from build123d import *

# Parameters (mm, degrees)
SKETCH1_W           = 50
SKETCH1_H           = 50
BOSS_EXTRUDE1_DEPTH = 0.8
FILLET1_R           = 5
SKETCH2_R           = 2
CUT_EXTRUDE1_DEPTH  = 36.364388868
SKETCH3_R           = 19.807187389
BOSS_EXTRUDE2_DEPTH = 1.5
SKETCH4_R           = 17.5
CUT_EXTRUDE2_DEPTH  = 1.5
SKETCH6_R           = 10
CUT_EXTRUDE3_DEPTH  = 36.387144558


with BuildPart() as part:
    # Sketch1 → Boss-Extrude1 (new body)
    with BuildSketch(Plane.XY):
        Rectangle(SKETCH1_W, SKETCH1_H)
    extrude(amount=BOSS_EXTRUDE1_DEPTH)

    # Fillet1
    fillet1_edges = [part.edges().sort_by_distance(p)[0] for p in [
        (25, -25, 0.4),
        (-25, -25, 0.4),
        (-25, 25, 0.4),
        (25, 25, 0.4),
    ]]
    fillet(fillet1_edges, radius=FILLET1_R)

    # Sketch2 → Cut-Extrude1 (cut, through all)
    with BuildSketch(Plane(origin=(0, 0, 0), x_dir=(-1, 0, 0), z_dir=(0, 0, -1))):
        with Locations((-20, 20)):
            Circle(SKETCH2_R)
        with Locations((20, 20)):
            Circle(SKETCH2_R)
        with Locations((20, -20)):
            Circle(SKETCH2_R)
        with Locations((-20, -20)):
            Circle(SKETCH2_R)
    extrude(amount=-CUT_EXTRUDE1_DEPTH, mode=Mode.SUBTRACT)

    # Sketch3 → Boss-Extrude2 (add)
    with BuildSketch(Plane(origin=(0, 0, 0), x_dir=(-1, 0, 0), z_dir=(0, 0, -1))):
        with Locations(Location((0, 0, 0), (0, 0, 180))):
            Circle(SKETCH3_R)
    extrude(amount=BOSS_EXTRUDE2_DEPTH)

    # Sketch4 → Cut-Extrude2 (cut)
    with BuildSketch(Plane(origin=(0, 0, -1.5), x_dir=(-1, 0, 0), z_dir=(0, 0, -1))):
        Circle(SKETCH4_R)
    extrude(amount=-CUT_EXTRUDE2_DEPTH, mode=Mode.SUBTRACT)

    # Sketch6 → Cut-Extrude3 (cut, through all)
    with BuildSketch(Plane(origin=(0, 0, 0), x_dir=(-1, 0, 0), z_dir=(0, 0, -1))):
        Circle(SKETCH6_R)
    extrude(amount=-CUT_EXTRUDE3_DEPTH, mode=Mode.SUBTRACT)


solid = part.part
Build history of the part. All positions in model axes, mm. A direction names the side the tool comes from. Coordinates: 2 decimals unless noted, no trailing zeros. Order: outer loops, then holes, each group sorted by start corner. A loop starts at its lowest first (then second) coordinate and runs counter-clockwise, first axis right, second up. Notation, with made-up numbers: M -22,-10.5 L 17,-10.5 A24 cw 17,3.5 Z; hole C -39.5,-12.75 d11. An arc over 180 degrees is marked long. One line per question, with ' | ' between items. Start each with the question number.
Q1. Two-plate mould, pull along Y, no slides. Class faces 1 (the face through (-19.74, 21.983, 0.394)), 2 (the face through (23.5, -23.57, 0.41)), 3 (the face through (-23.57, 23.5, 0.41)): +Y half, -Y half, draft (parallel to the pull), parting line (faces both ways), or undercut.
Q2. Saw through at A-A (x = 0). List the corners of the cut face in (y, z).
Q3. Flat gauge pins, fed straight in: pin 1 Ø2.5 at (x, y) = (20, -20) entering from -Z; pin 2 Ø10.5 at (x, y) = (-8, 5.5) entering from -Z; pin 3 Ø25 at (x, y) = (1.5, 8.5) entering from -Z. Where does each tip first touch, or does it go through?
Q4. 3-axis set-ups, long thin cutter, end or side, ignore diameter. For faces 4 (the face through (13.887, -10.648, -0.76)), 5 (the face through (-23.57, -23.5, 0.41)): which of +Z, -Z, +X, -X, +Y, -Y reach the whole face in a straight line?
Q5. Saw through at D-D (x = 12). List the corners of the cut face in (y, z), then the cut area to 3 significant figures.
Q6. Saw through at C-C (y = 21). List the corners of the cut face in (x, z), then the cut area to 3 significant figures.
Q7. Probe L1, parallel to Y at x = 20, z = 0.5; L2, parallel to X at y = -0.5, z = 0.2; L3, parallel to Z at x = 12, y = 8.5. List the from-to ranges inside material, lowest first. Write a range as from..to.
Check values:
1) face 1: undercut | face 2: -Y half | face 3: +Y half
2) outline: M -25,0 L -19.81,0 L -19.81,-1.5 L -17.5,-1.5 L -17.5,0 L -10,0 L -10,0.8 L -25,0.8 Z; M 10,0 L 17.5,0 L 17.5,-1.5 L 19.81,-1.5 L 19.81,0 L 25,0 L 25,0.8 L 10,0.8 Z
3) pin 1: passes through | pin 2: stops at z = 0 | pin 3: stops at z = -1.5
4) face 4: -Z | face 5: +Z, -Z, -X, -Y
5) outline: M -25,0 L -15.76,0 L -15.76,-1.5 L -12.74,-1.5 L -12.74,0 L 12.74,0 L 12.74,-1.5 L 15.76,-1.5 L 15.76,0 L 25,0 L 25,0.8 L -25,0.8 Z | area: 49.1 mm2
6) outline: M -24.9,0 L -21.73,0 L -21.73,0.8 L -24.9,0.8 Z; M -18.27,0 L 18.27,0 L 18.27,0.8 L -18.27,0.8 Z; M 21.73,0 L 24.9,0 L 24.9,0.8 L 21.73,0.8 Z | area: 34.3 mm2
7) L1: y = -25..-22, -18..18, 22..25 | L2: x = -25..-9.99, 9.99..25 | L3: z = 0..0.8
